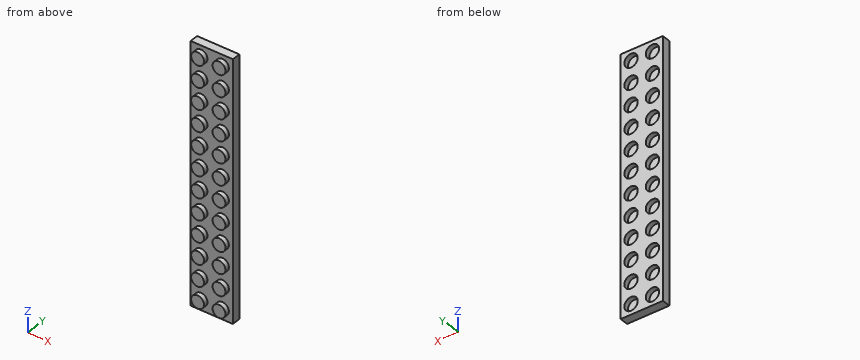
from build123d import *

# Parameters (mm, degrees)
SKETCH_1_W          = 15.8
SKETCH_1_H          = 95.8
EXTRUDE_1_DEPTH     = 3.2
SKETCH_2_R          = 2.4
EXTRUDE_3_DEPTH     = 1.7
SKETCH_3_R          = 2.5
CUT_EXTRUDE_1_DEPTH = 1.8


with BuildPart() as part:
    # Эскиз1 → Бобышка-Вытянуть1 (new body)
    with BuildSketch(Plane(origin=(0, 0, 0), x_dir=(1, 0, 0), z_dir=(0, 1, 0))):
        Rectangle(SKETCH_1_W, SKETCH_1_H)
    extrude(amount=EXTRUDE_1_DEPTH)

    # Эскиз2 → Бобышка-Вытянуть3 (add)
    with BuildSketch(Plane.XZ):
        with Locations(Location((-4, -44, 0), (0, 0, 90))):
            Circle(SKETCH_2_R)
        with Locations(Location((4, -44, 0), (0, 0, 90))):
            Circle(SKETCH_2_R)
        with Locations(Location((4, -36, 0), (0, 0, 90))):
            Circle(SKETCH_2_R)
        with Locations(Location((4, -28, 0), (0, 0, 90))):
            Circle(SKETCH_2_R)
        with Locations(Location((4, -20, 0), (0, 0, 90))):
            Circle(SKETCH_2_R)
        with Locations(Location((4, -12, 0), (0, 0, 90))):
            Circle(SKETCH_2_R)
        with Locations(Location((4, -4, 0), (0, 0, 90))):
            Circle(SKETCH_2_R)
        with Locations(Location((4, 4, 0), (0, 0, 90))):
            Circle(SKETCH_2_R)
        with Locations(Location((4, 12, 0), (0, 0, 90))):
            Circle(SKETCH_2_R)
        with Locations(Location((4, 20, 0), (0, 0, 90))):
            Circle(SKETCH_2_R)
        with Locations(Location((4, 28, 0), (0, 0, 90))):
            Circle(SKETCH_2_R)
        with Locations(Location((4, 36, 0), (0, 0, 90))):
            Circle(SKETCH_2_R)
        with Locations(Location((4, 44, 0), (0, 0, 90))):
            Circle(SKETCH_2_R)
        with Locations(Location((-4, -36, 0), (0, 0, 90))):
            Circle(SKETCH_2_R)
        with Locations(Location((-4, -28, 0), (0, 0, 90))):
            Circle(SKETCH_2_R)
        with Locations(Location((-4, -20, 0), (0, 0, 90))):
            Circle(SKETCH_2_R)
        with Locations(Location((-4, -12, 0), (0, 0, 90))):
            Circle(SKETCH_2_R)
        with Locations(Location((-4, -4, 0), (0, 0, 90))):
            Circle(SKETCH_2_R)
        with Locations(Location((-4, 4, 0), (0, 0, 90))):
            Circle(SKETCH_2_R)
        with Locations(Location((-4, 12, 0), (0, 0, 90))):
            Circle(SKETCH_2_R)
        with Locations(Location((-4, 20, 0), (0, 0, 90))):
            Circle(SKETCH_2_R)
        with Locations(Location((-4, 28, 0), (0, 0, 90))):
            Circle(SKETCH_2_R)
        with Locations(Location((-4, 36, 0), (0, 0, 90))):
            Circle(SKETCH_2_R)
        with Locations(Location((-4, 44, 0), (0, 0, 90))):
            Circle(SKETCH_2_R)
    extrude(amount=EXTRUDE_3_DEPTH)

    # Эскиз3 → Вырез-Вытянуть1 (cut)
    with BuildSketch(Plane(origin=(0, 3.2, 0), x_dir=(1, 0, 0), z_dir=(0, 1, 0))):
        with Locations(Location((-4, -44, 0), (0, 0, 270))):
            Circle(SKETCH_3_R)
        with Locations(Location((4, -44, 0), (0, 0, 270))):
            Circle(SKETCH_3_R)
        with Locations(Location((4, -36, 0), (0, 0, 270))):
            Circle(SKETCH_3_R)
        with Locations(Location((4, -28, 0), (0, 0, 270))):
            Circle(SKETCH_3_R)
        with Locations(Location((4, -20, 0), (0, 0, 270))):
            Circle(SKETCH_3_R)
        with Locations(Location((4, -12, 0), (0, 0, 270))):
            Circle(SKETCH_3_R)
        with Locations(Location((4, -4, 0), (0, 0, 270))):
            Circle(SKETCH_3_R)
        with Locations(Location((4, 4, 0), (0, 0, 270))):
            Circle(SKETCH_3_R)
        with Locations(Location((4, 12, 0), (0, 0, 270))):
            Circle(SKETCH_3_R)
        with Locations(Location((4, 20, 0), (0, 0, 270))):
            Circle(SKETCH_3_R)
        with Locations(Location((4, 28, 0), (0, 0, 270))):
            Circle(SKETCH_3_R)
        with Locations(Location((4, 36, 0), (0, 0, 270))):
            Circle(SKETCH_3_R)
        with Locations(Location((4, 44, 0), (0, 0, 270))):
            Circle(SKETCH_3_R)
        with Locations(Location((-4, -36, 0), (0, 0, 270))):
            Circle(SKETCH_3_R)
        with Locations(Location((-4, -28, 0), (0, 0, 270))):
            Circle(SKETCH_3_R)
        with Locations(Location((-4, -20, 0), (0, 0, 270))):
            Circle(SKETCH_3_R)
        with Locations(Location((-4, -12, 0), (0, 0, 270))):
            Circle(SKETCH_3_R)
        with Locations(Location((-4, -4, 0), (0, 0, 270))):
            Circle(SKETCH_3_R)
        with Locations(Location((-4, 4, 0), (0, 0, 270))):
            Circle(SKETCH_3_R)
        with Locations(Location((-4, 12, 0), (0, 0, 270))):
            Circle(SKETCH_3_R)
        with Locations(Location((-4, 20, 0), (0, 0, 270))):
            Circle(SKETCH_3_R)
        with Locations(Location((-4, 28, 0), (0, 0, 270))):
            Circle(SKETCH_3_R)
        with Locations(Location((-4, 36, 0), (0, 0, 270))):
            Circle(SKETCH_3_R)
        with Locations(Location((-4, 44, 0), (0, 0, 270))):
            Circle(SKETCH_3_R)
    extrude(amount=-CUT_EXTRUDE_1_DEPTH, mode=Mode.SUBTRACT)


solid = part.part
Could you check a few things on this model? Use its own coordinates, in mm. Coordinates: 2 decimals unless noted, no trailing zeros. Loops run counter-clockwise (first coordinate to the right, second up) from the corner with the lowest first, then second, coordinate; pieces in that order, holes last. Notation, with made-up numbers: (11.25, 13.25) -> (29.25, 13.25) arc R7 ccw to (29.25, 17.25) -> close; hole circle Ø4 at (7.5, 59.5). An arc over 180 degrees is marked (long way). Answer in a Markdown table with one row per item.
(1) Imagine slicing it at B-B (z = -44). List the corners of the cut face in (x, y) for me.
Results found:
| item | result |
|---|---|
| outline | (-7.9, 0) -> (-6.4, 0) -> (-6.4, -1.7) -> (-1.6, -1.7) -> (-1.6, 0) -> (1.6, 0) -> (1.6, -1.7) -> (6.4, -1.7) -> (6.4, 0) -> (7.9, 0) -> (7.9, 3.2) -> (6.5, 3.2) -> (6.5, 1.4) -> (1.5, 1.4) -> (1.5, 3.2) -> (-1.5, 3.2) -> (-1.5, 1.4) -> (-6.5, 1.4) -> (-6.5, 3.2) -> (-7.9, 3.2) -> close |
(2) If I drill on probe 1 along X at (y, z) = (2.1, 36); probe 2 along X at (y, z) = (2.1, -10.5); probe 3 along Y at (x, z) = (1.75, 7), over which ranges is the centre line in solid material (lowest first)?
Results found:
| item | result |
|---|---|
| probe 1 | x = -7.9 to -6.5, -1.5 to 1.5, 6.5 to 7.9 |
| probe 2 | x = -7.9 to -6, -2 to 2, 6 to 7.9 |
| probe 3 | y = 0 to 3.2 |
(3) Will these pins go through, and if not, where does the flat tip stop? pin 1 Ø6 at (x, z) = (-4, -12) entering from +Y; pin 2 Ø2.5 at (x, z) = (-4, 13) entering from +Y.
Results found:
| item | result |
|---|---|
| pin 1 | stops at y = 3.2 |
| pin 2 | stops at y = 1.4 |
(4) Imagine slicing it at A-A (y = 2.45). Give the number of separate pieces and of enclosed holes in the cut face, plus the area to 3 significant figures.
Results found:
| item | result |
|---|---|
| separate pieces | 1 |
| enclosed holes | 24 |
| area | 1,040 mm^2 |
(5) Imagine slicing it at D-D (z = 36.5). List the corners of the cut face in (x, y) for me, plus the area to 3 significant figures.
Results found:
| item | result |
|---|---|
| outline | (-7.9, 0) -> (-6.35, 0) -> (-6.35, -1.7) -> (-1.65, -1.7) -> (-1.65, 0) -> (1.65, 0) -> (1.65, -1.7) -> (6.35, -1.7) -> (6.35, 0) -> (7.9, 0) -> (7.9, 3.2) -> (6.45, 3.2) -> (6.45, 1.4) -> (1.55, 1.4) -> (1.55, 3.2) -> (-1.55, 3.2) -> (-1.55, 1.4) -> (-6.45, 1.4) -> (-6.45, 3.2) -> (-7.9, 3.2) -> close |
| area | 48.9 mm^2 |
(6) Imagine slicing it at C-C (x = -0.5). List the corners of the cut face in (y, z) for me, plus the area to 3 significant figures.
Results found:
| item | result |
|---|---|
| outline | (0, -47.9) -> (3.2, -47.9) -> (3.2, 47.9) -> (0, 47.9) -> close |
| area | 307 mm^2 |
